Part model, mm, in its own coordinate system. A direction names the side the tool comes from. Round coordinates to 2 decimals unless told otherwise and drop trailing zeros. Write each loop counter-clockwise with the first axis right and the second up, starting at its lowest first coordinate (ties: lowest second). Pieces come first, ordered by that corner, then holes. Notation, with made-up numbers: M 39,77.5 L 86,77.5 A15 ccw 86,102.5 Z; hole C 63.25,16.5 d2. An arc over 180 degrees is marked long. Use one line per item in the form item = value. Start each with the question number.
Item 1: Flat gauge pins, fed straight in: pin 1 Ø2 at (y, z) = (32.5, -0.5) entering from -X; pin 2 Ø5 at (x, y) = (8, 12) entering from -Z; pin 3 Ø2.5 at (x, y) = (6.5, 6) entering from +Z; pin 4 Ø5.5 at (x, z) = (6.5, -5) entering from +Y. Where does each tip first touch, or does it go through?
Item 2: Cut at D-D, the plane x = 4. Give the cut face in (y, z), then the cut area to 3 significant figures.
Item 3: Mould opens along X. For faces 1 (the face through (9.8, 25, 2)), 2 (the face through (13, 14, 1)), 3 (the face through (6, -3.2, -3)) say: +X half, -X half, draft (parallel to the pull), parting line (faces both ways), or undercut.
Item 4: Probe L1, parallel to Y at x = 6.5, z = 2.55; L2, parallel to X at y = -2.1, z = -5; L3, parallel to Y at x = 7, z = 1.25. List the from-to ranges inside material, lowest first.
Item 5: Cut at C-C, the plane z = 2. Give the cut face in (x, y).
Item 6: Which spindle directions (+Z, -Z, +X, -X, +Y, -Y) get a long thin tool onto all of the face, cutting with end or side? Do faces 4 (the face through (9.2, 37.43, 1.58)), 5 (the face through (2, 24, 0)), 6 (the face through (6.6, -1.6, -11.5)). Say none if no direction does.
Item 7: Cut at A-A, the plane x = 6.5. Give the cut face in (y, z), then the cut area to 3 significant figures.
Item 8: Cut at B-B, the plane y = 33.5. Give the cut face in (x, z).
from build123d import *

# Parameters (mm, degrees)
SKETCH1_R           = 1.4
BOSS_EXTRUDE1_DEPTH = 3.2
SKETCH2_R           = 1.65
BOSS_EXTRUDE3_DEPTH = 3.2
BOSS_EXTRUDE4_DEPTH = 2
LPATTERN1_COUNT     = 2
LPATTERN1_PITCH     = 11
CUT_EXTRUDE1_DEPTH  = 50.633657935


with BuildPart() as part:
    # Sketch1 → Boss-Extrude1 (new body)
    with BuildSketch(Plane.XY):
        with BuildLine():
            Line((0, 0), (13, 0))
            Line((13, 0), (13, 40.5))
            ThreePointArc((13, 40.5), (11.242640687, 44.742640687), (7, 46.5))
            Line((7, 46.5), (6, 46.5))
            ThreePointArc((6, 46.5), (1.757359313, 44.742640687), (0, 40.5))
            Line((0, 40.5), (0, 0))
        make_face()
        with Locations((6.5, 6)):
            Circle(SKETCH1_R, mode=Mode.SUBTRACT)
        with Locations((6.5, 43)):
            Circle(SKETCH1_R, mode=Mode.SUBTRACT)
    extrude(amount=BOSS_EXTRUDE1_DEPTH)

    # Sketch2 → Boss-Extrude3 (add)
    with BuildSketch(Plane(origin=(0, 0, 0), x_dir=(1, 0, 0), z_dir=(0, 1, 0))):
        with BuildLine():
            Line((0, 5), (0, -3.2))
            Line((0, -3.2), (13, -3.2))
            Line((13, -3.2), (13, 5))
            ThreePointArc((13, 5), (6.5, 11.5), (0, 5))
        make_face()
        with Locations(Location((6.5, 5, 0), (0, 0, 270))):
            Circle(SKETCH2_R, mode=Mode.SUBTRACT)
    extrude(amount=-BOSS_EXTRUDE3_DEPTH)

    # Sketch3 → Boss-Extrude4 (add)
    with BuildSketch(Plane(origin=(0, 0, 0), x_dir=(0, 0, -1), z_dir=(1, 0, 0))):
        Polygon((0, 0), (5, 0), (0, 8), align=None)
    boss_extrude4 = extrude(amount=BOSS_EXTRUDE4_DEPTH)

    # LPattern1: Boss-Extrude4 ×2
    with Locations(*[(i * LPATTERN1_PITCH, 0, 0) for i in range(1, LPATTERN1_COUNT)]):
        add(boss_extrude4)

    # Sketch4 → Cut-Extrude1 (cut, through all)
    with BuildSketch(Plane.XY):
        with BuildLine():
            Line((5.2, 38), (7.8, 38))
            ThreePointArc((7.8, 38), (9.214213562, 37.414213562), (9.8, 36))
            Line((9.8, 36), (9.8, 13))
            ThreePointArc((9.8, 13), (9.214213562, 11.585786438), (7.8, 11))
            Line((7.8, 11), (5.2, 11))
            ThreePointArc((5.2, 11), (3.785786438, 11.585786438), (3.2, 13))
            Line((3.2, 13), (3.2, 36))
            ThreePointArc((3.2, 36), (3.785786438, 37.414213562), (5.2, 38))
        make_face()
    extrude(amount=CUT_EXTRUDE1_DEPTH, mode=Mode.SUBTRACT)


solid = part.part
Model answer:
q1.pin_1 = 0
q1.pin_2 = 0
q1.pin_3 = through
q1.pin_4 = 0
q2.outline = M -3.2,-11 L 0,-11 L 0,0 L 11.4,0 L 11.4,3.2 L -3.2,3.2 Z; M 37.6,0 L 46.16,0 L 46.16,3.2 L 37.6,3.2 Z
q2.area = 109 mm²
q3.face_1 = undercut
q3.face_2 = +X half
q3.face_3 = draft
q4.L1 = -3.2 to 4.6, 7.4 to 11, 38 to 41.6, 44.4 to 46.5
q4.L2 = 0 to 4.85, 8.15 to 13
q4.L3 = -3.2 to 4.69, 7.31 to 11, 38 to 41.69, 44.31 to 46.5
q5.outline = M 0,-3.2 L 13,-3.2 L 13,40.5 A6 ccw 7,46.5 L 6,46.5 A6 ccw 0,40.5 Z; hole M 3.2,13 A2 ccw 5.2,11 L 7.8,11 A2 ccw 9.8,13 L 9.8,36 A2 ccw 7.8,38 L 5.2,38 A2 ccw 3.2,36 Z; hole C 6.5,6 d2.8; hole C 6.5,43 d2.8
q6.face_4 = +Z, -Z
q6.face_5 = -Z, +Y
q6.face_6 = -Z, +Y, -Y
q7.outline = M -3.2,-11.5 L 0,-11.5 L 0,-6.65 L -3.2,-6.65 Z; M -3.2,-3.35 L 0,-3.35 L 0,0 L 4.6,0 L 4.6,3.2 L -3.2,3.2 Z; M 7.4,0 L 11,0 L 11,3.2 L 7.4,3.2 Z; M 38,0 L 41.6,0 L 41.6,3.2 L 38,3.2 Z; M 44.4,0 L 46.5,0 L 46.5,3.2 L 44.4,3.2 Z
q7.area = 81.0 mm²
q8.outline = M 0,0 L 3.2,0 L 3.2,3.2 L 0,3.2 Z; M 9.8,0 L 13,0 L 13,3.2 L 9.8,3.2 Z
